Here's how the part is built. I have some questions about the finished solid (model axes, mm). A direction names the side the tool comes from. Give positions to 0.01 mm unless a question says otherwise; leave off trailing zeros. Order: outer loops, then holes, each group sorted by start corner. A loop starts at its lowest first (then second) coordinate and runs counter-clockwise, first axis right, second up.
from build123d import *

# Parameters (mm, degrees)
SKETCH_1_W          = 40
SKETCH_1_H          = 100
SKETCH_1_R          = 1.6
SKETCH_1_R_2        = 3
EXTRUDE_1_DEPTH     = 3
SKETCH_2_W          = 20
SKETCH_2_H          = 15
CUT_EXTRUDE_1_DEPTH = 108.745069493
CHAMFER_1_SIZE      = 3
SKETCH_3_W          = 25
SKETCH_3_H          = 50
CUT_EXTRUDE_2_DEPTH = 108.745069493
CHAMFER_2_SIZE      = 8


with BuildPart() as part:
    # ｽｹｯﾁ1 → ﾎﾞｽ - 押し出し1 (new body)
    with BuildSketch(Plane.XY):
        with Locations((20, 50)):
            Rectangle(SKETCH_1_W, SKETCH_1_H)
        with Locations((5, 95)):
            Circle(SKETCH_1_R, mode=Mode.SUBTRACT)
        with Locations((35, 95)):
            Circle(SKETCH_1_R, mode=Mode.SUBTRACT)
        with Locations((5, 80)):
            Circle(SKETCH_1_R_2, mode=Mode.SUBTRACT)
        with Locations((35, 70)):
            Circle(SKETCH_1_R_2, mode=Mode.SUBTRACT)
        with Locations((5, 20)):
            Circle(SKETCH_1_R_2, mode=Mode.SUBTRACT)
        with Locations((35, 30)):
            Circle(SKETCH_1_R_2, mode=Mode.SUBTRACT)
        with Locations((5, 5)):
            Circle(SKETCH_1_R, mode=Mode.SUBTRACT)
        with Locations((35, 5)):
            Circle(SKETCH_1_R, mode=Mode.SUBTRACT)
    extrude(amount=EXTRUDE_1_DEPTH)

    # ｽｹｯﾁ2 → ｶｯﾄ - 押し出し1 (cut, through all)
    with BuildSketch(Plane.XY.offset(3)):
        with Locations((20, 92.5)):
            Rectangle(SKETCH_2_W, SKETCH_2_H)
        with Locations((20, 7.5)):
            Rectangle(SKETCH_2_W, SKETCH_2_H)
    extrude(amount=-CUT_EXTRUDE_1_DEPTH, mode=Mode.SUBTRACT)

    # 面取り1
    chamfer_1_edges = [part.edges().sort_by_distance(p)[0] for p in [
        (10, 85, 1.5),
        (30, 85, 1.5),
        (10, 15, 1.5),
        (30, 15, 1.5),
    ]]
    chamfer(chamfer_1_edges, length=CHAMFER_1_SIZE)

    # ｽｹｯﾁ3 → ｶｯﾄ - 押し出し2 (cut, through all)
    with BuildSketch(Plane(origin=(0, 0, 0), x_dir=(-1, 0, 0), z_dir=(0, 0, -1))):
        with Locations((-12.5, 50)):
            Rectangle(SKETCH_3_W, SKETCH_3_H)
    extrude(amount=-CUT_EXTRUDE_2_DEPTH, mode=Mode.SUBTRACT)

    # 面取り2
    chamfer_2_edges = [part.edges().sort_by_distance(p)[0] for p in [
        (25, 25, 1.5),
        (25, 75, 1.5),
    ]]
    chamfer(chamfer_2_edges, length=CHAMFER_2_SIZE)


solid = part.part
Q1. For faces 1 (the face through (20, 85, 2)), 2 (the face through (21, 71, 1)), 3 (the face through (28, 14, 2)), which set-ups out of +Z, -Z, +X, -X, +Y, -Y let a thin tool reach every point of the face, with its end or its side?
Filled sheet:
face 1: +Z, -Z, +Y
face 2: +Z, -Z, -X
face 3: +Z, -Z, -Y
Q2. I'm going to push a flat-ended pin straight in: P1, Ø1.5, axis at x = 20, z = 2, coming from the +Y side. Where does the tip first touch, or does it pass through?
Filled sheet:
P1: stops at y = 85
Q3. I need wall thicknesses on L1, parallel to X at y = 95, z = 0.8; L2, parallel to Y at x = 5, z = 2.25; L3, parallel to Y at x = 19, z = 1.65. Which ranges of each line are inside material? Lowest first, please.
Filled sheet:
L1: x = 0 to 3.4, 6.6 to 10, 30 to 33.4, 36.6 to 40
L2: y = 0 to 3.4, 6.6 to 17, 23 to 25, 75 to 77, 83 to 93.4, 96.6 to 100
L3: y = 15 to 27, 73 to 85
Q4. If we section it at D-D on y = 30: List the corners of the cut face in (x, z) for me.
Filled sheet:
outline: (22, 0) - (32, 0) - (32, 3) - (22, 3) - close; (38, 0) - (40, 0) - (40, 3) - (38, 3) - close
Q5. Thinking about a two-plate mould opening in Y: for faces 4 (the face through (21, 29, 1)), 5 (the face through (5, 0, 1)), 6 (the face through (29, 51, 3)), which applies, released by +Y, released by -Y, zero draft, split by the parting line, or undercut?
Filled sheet:
face 4: undercut
face 5: released by -Y
face 6: zero draft
Q6. If we section it at C-C on z = 1.15: Give the number of separate pieces and of enclosed holes in the cut face, plus the area to 3 significant figures.
Filled sheet:
separate pieces: 1
enclosed holes: 8
area: 2,090 mm2
Q7. If we section it at B-B on x = 22.5: List the corners of the cut face in (y, z) for me, plus the area to 3 significant figures.
Filled sheet:
outline: (15, 0) - (30.5, 0) - (30.5, 3) - (15, 3) - close; (69.5, 0) - (85, 0) - (85, 3) - (69.5, 3) - close
area: 93.0 mm2
Q8. If we section it at A-A on y = 5: List the corners of the cut face in (x, z) for me, plus the area to 3 significant figures.
Filled sheet:
outline: (0, 0) - (3.4, 0) - (3.4, 3) - (0, 3) - close; (6.6, 0) - (10, 0) - (10, 3) - (6.6, 3) - close; (30, 0) - (33.4, 0) - (33.4, 3) - (30, 3) - close; (36.6, 0) - (40, 0) - (40, 3) - (36.6, 3) - close
area: 40.8 mm2
